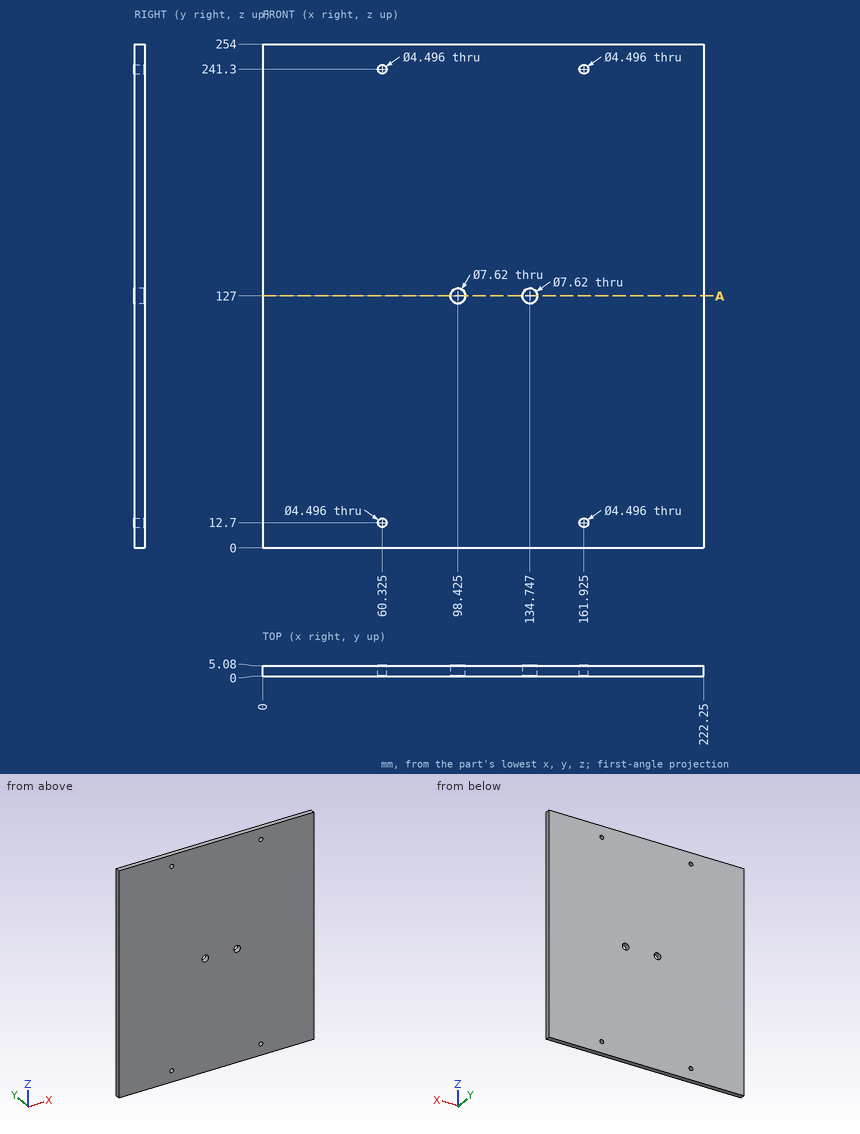
Job drawing, mm, ordinate dimensions from the low corner. One solid piece. Give positions to 0.01 mm unless a question says otherwise; leave off trailing zeros. Write each loop counter-clockwise with the first axis right and the second up, starting at its lowest first coordinate (ties: lowest second). Pieces come first, ordered by that corner, then holes. Notation, with made-up numbers: (82.5, 18) - (86.5, 18) arc R32 ccw to (86.5, 51) - close; hole circle Ø9 at (31.5, 71.5). An arc over 180 degrees is marked (long way). Answer as CSV lines item,"result".
1. Pin check, flat tip, straight feed: pin 1 (4 mm diameter, centred on x = 60.325, z = 241.3, fed in from -Y). Stop position of the tip, or through.
Responses:
pin 1,"passes through"
2. Band-saw the part on A-A (z = 127). Write the cut outline in (x, y) (3 decimals).
Responses:
outline,"(0, 0) - (94.615, 0) - (94.615, 5.08) - (0, 5.08) - close; (102.235, 0) - (130.937, 0) - (130.937, 5.08) - (102.235, 5.08) - close; (138.557, 0) - (222.25, 0) - (222.25, 5.08) - (138.557, 5.08) - close"
3. Drill centre lines: L1, parallel to X at y = 1.35, z = 127 (3 decimals); L2, parallel to X at y = 2.05, z = 241.3; L3, parallel to Z at x = 135, y = 0.7. Where is each one in solid material? Low to high. Write a range as [from, to].
Responses:
L1,"x = [0, 94.615], [102.235, 130.937], [138.557, 222.25]"
L2,"x = [0, 58.08], [62.57, 159.68], [164.17, 222.25]"
L3,"z = [0, 123.2], [130.8, 254]"
